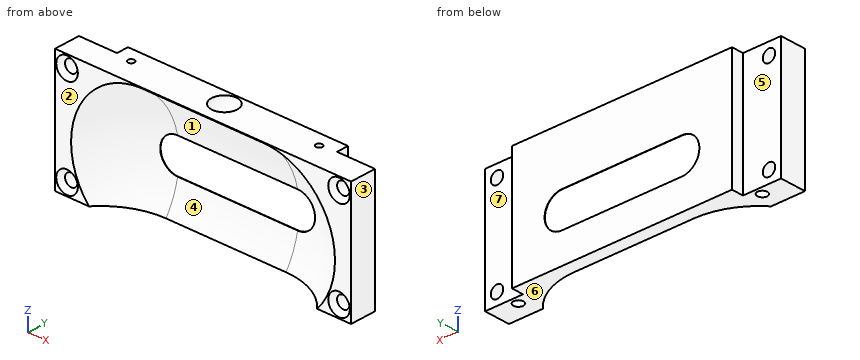
from build123d import *

# Parameters (mm, degrees)
SKETCH1_W                                       = 74
SKETCH1_H                                       = 30
BOSS_EXTRUDE1_DEPTH                             = 9.5
SKETCH2_W                                       = 9.5
SKETCH2_H                                       = 30
CUT_EXTRUDE1_DEPTH                              = 3
CSK_FOR_M3_FLAT_HEAD_MACHINE_SCREW1_D           = 3.1
CSK_FOR_M3_FLAT_HEAD_MACHINE_SCREW1_CSINK_D     = 5.4
CSK_FOR_M3_FLAT_HEAD_MACHINE_SCREW1_CSINK_ANGLE = 90
SKETCH14_W                                      = 30
SKETCH14_H                                      = 21.35
SKETCH21_R                                      = 0.8
CUT_EXTRUDE2_DEPTH                              = 6
TAP_DRILL_FOR_M3X0_5_TAP1_D                     = 2.5
TAP_DRILL_FOR_M3X0_5_TAP1_DEPTH                 = 4.5
TAP_DRILL_FOR_M3X0_5_TAP1_TIP                   = 0.751075774
CUT_EXTRUDE3_DEPTH                              = 10


with BuildPart() as part:
    # Sketch1 → Boss-Extrude1 (new body)
    with BuildSketch(Plane(origin=(0, 0, 0), x_dir=(1, 0, 0), z_dir=(0, 1, 0))):
        with Locations((37, 15)):
            Rectangle(SKETCH1_W, SKETCH1_H)
    extrude(amount=BOSS_EXTRUDE1_DEPTH)

    # Sketch2 → Cut-Extrude1 (cut)
    with BuildSketch(Plane(origin=(0, 9.5, 0), x_dir=(1, 0, 0), z_dir=(0, 1, 0))):
        with Locations((69.25, 15)):
            Rectangle(SKETCH2_W, SKETCH2_H)
        with Locations((4.75, 15)):
            Rectangle(SKETCH2_W, SKETCH2_H)
    extrude(amount=-CUT_EXTRUDE1_DEPTH, mode=Mode.SUBTRACT)

    # CSK for M3 Flat Head Machine Screw1 (through all)
    with Locations(Plane(origin=(3, 0, -3), x_dir=(0, 0, -1), z_dir=(0, -1, 0))):
        with Locations((0, 0), (24, 0), (24, 68), (0, 68)):
            CounterSinkHole(CSK_FOR_M3_FLAT_HEAD_MACHINE_SCREW1_D / 2, CSK_FOR_M3_FLAT_HEAD_MACHINE_SCREW1_CSINK_D / 2, counter_sink_angle=CSK_FOR_M3_FLAT_HEAD_MACHINE_SCREW1_CSINK_ANGLE)

    # Sketch12 → Cut-Revolve5 (revolve, cut)
    with BuildSketch(Plane(origin=(0, -11.5, 0), x_dir=(-1, 0, 0), z_dir=(0, -1, 0))):
        with BuildLine():
            Line((-52, -3.2), (-52, 39.5))
            ThreePointArc((-52, 39.5), (-73.35, 18.15), (-52, -3.2))
        make_face()
    revolve(axis=Axis((52, -11.5, 3.2), (0, 0, -1)), mode=Mode.SUBTRACT)

    # Sketch12<8> → Cut-Revolve6 (revolve, cut)
    with BuildSketch(Plane(origin=(0, -11.5, 0), x_dir=(-1, 0, 0), z_dir=(0, -1, 0))):
        with BuildLine():
            Line((-22, -3.2), (-22, 39.5))
            ThreePointArc((-22, 39.5), (-0.65, 18.15), (-22, -3.2))
        make_face()
    revolve(axis=Axis((22, -11.5, 3.2), (0, 0, -1)), mode=Mode.SUBTRACT)

    # Sketch14 → Cut-Revolve7 (revolve, cut)
    with BuildSketch(Plane(origin=(0, -11.5, 0), x_dir=(-1, 0, 0), z_dir=(0, -1, 0))):
        with Locations((-37, 28.825)):
            Rectangle(SKETCH14_W, SKETCH14_H)
    revolve(axis=Axis((52, -11.5, -18.15), (-1, 0, 0)), mode=Mode.SUBTRACT)

    # Sketch20 one side → Cut-Revolve8 (revolve, cut)
    with BuildSketch(Plane.XY):
        with BuildLine():
            ThreePointArc((37, 9), (33.8, 5.8), (37, 2.6))
            Line((37, 2.6), (37, 9))
        make_face()
    revolve(axis=Axis((37, 9, 0), (0, -1, 0)), mode=Mode.SUBTRACT)

    # Sketch21 → Cut-Extrude2 (cut)
    with BuildSketch(Plane.XY):
        with Locations((13.5, 6)):
            Circle(SKETCH21_R)
        with Locations((60.5, 6)):
            Circle(SKETCH21_R)
    extrude(amount=-CUT_EXTRUDE2_DEPTH, mode=Mode.SUBTRACT)

    # Tap Drill for M3x0.5 Tap1
    with Locations(Plane(origin=(6.5, 4.5, -30), x_dir=(-1, 0, 0), z_dir=(0, 0, -1))):
        with Locations((0, 0), (-61, 0)):
            Hole(TAP_DRILL_FOR_M3X0_5_TAP1_D / 2, depth=TAP_DRILL_FOR_M3X0_5_TAP1_DEPTH)
            with Locations((0, 0, -(TAP_DRILL_FOR_M3X0_5_TAP1_DEPTH + TAP_DRILL_FOR_M3X0_5_TAP1_TIP / 2))):  # 118° drill point
                Cone(0, TAP_DRILL_FOR_M3X0_5_TAP1_D / 2, TAP_DRILL_FOR_M3X0_5_TAP1_TIP, mode=Mode.SUBTRACT)

    # Sketch26 → Cut-Extrude3 (cut)
    with BuildSketch(Plane(origin=(0, 9.5, 0), x_dir=(1, 0, 0), z_dir=(0, 1, 0))):
        with BuildLine():
            Line((52, 13.8), (22, 13.8))
            ThreePointArc((22, 13.8), (17.65, 18.15), (22, 22.5))
            Line((22, 22.5), (52, 22.5))
            ThreePointArc((52, 22.5), (56.35, 18.15), (52, 13.8))
        make_face()
    extrude(amount=-CUT_EXTRUDE3_DEPTH, mode=Mode.SUBTRACT)


solid = part.part
Part model, mm, in its own coordinate system. Face numbers are marked on the shaded views. A direction names the side the tool comes from. Give positions to 0.01 mm unless a question says otherwise; leave off trailing zeros. Order: outer loops, then holes, each group sorted by start corner. A loop starts at its lowest first (then second) coordinate and runs counter-clockwise, first axis right, second up. Notation, with made-up numbers: (24, -21.75) -> (78, -21.75) arc R12 ccw to (78, -2.75) -> close; hole circle Ø1 at (39.25, -18.75). An arc over 180 degrees is marked (long way). Use one line per item in the form item = value.
(1) Saw through at D-D (z = -9). Write the cut outline in (x, y).
Solution:
outline = (0, 0) -> (6.51, 0) arc R19.29 cw to (22, 7.79) -> (52, 7.79) arc R19.29 cw to (67.49, 0) -> (74, 0) -> (74, 6.5) -> (64.5, 6.5) -> (64.5, 9.5) -> (9.5, 9.5) -> (9.5, 6.5) -> (0, 6.5) -> close
(2) Flat gauge pins, fed straight in: P1, Ø4, axis at x = 3, z = -27, coming from the -Y side; P2, Ø1.3, axis at x = 61, y = 5.5, coming from the +Z side; P3, Ø1, axis at x = 35, z = -12.5, coming from the -Y side; P4, Ø10.5, axis at x = 70.5, z = -17, coming from the +Y side. Where does each tip first touch, or does it go through?
Solution:
P1 = 0.7
P2 = 0
P3 = 8.95
P4 = 6.5
(3) Pull direction X, two halves, no side cores. Call the marked faces 1, 2, 3 and 4: +X half, -X half, draft (parallel to the pull), parting line (faces both ways), or undercut.
Solution:
face_1 = undercut
face_2 = draft
face_3 = +X half
face_4 = undercut
(4) Drill centre lines: line 1 (Z direction, x = 3, y = 5.4); line 2 (Y direction, x = 67.5, z = -29); line 3 (X direction, y = 4.5, z = -27.5). Where is each one in solid material? Low to high. Write a range as from..to.
Solution:
line_1 = -30..-28.55, -25.45..-4.55, -1.45..0
line_2 = 0..3.25, 5.75..6.5
line_3 = 0..1.53, 4.47..5.25, 7.75..11.4, 62.6..66.25, 68.75..69.53, 72.47..74
(5) Tool access for the marked faces 5, 6 and 7: list every direction of +Z, -Z, +X, -X, +Y, -Y with a clear straight run to the whole face (end or side of a thin tool).
Solution:
face_5 = +Z, -Z, -X, +Y
face_6 = -Z, +X, -X, +Y, -Y
face_7 = +Z, -Z, +X, +Y
(6) Saw through at B-B (x = 71). Write the cut outline in (y, z), then the cut area to 3 significant figures.
Solution:
outline = (0, -30) -> (6.5, -30) -> (6.5, -28.55) -> (1.15, -28.55) -> (0, -29.7) -> close; (0, -24.3) -> (1.15, -25.45) -> (6.5, -25.45) -> (6.5, -4.55) -> (1.15, -4.55) -> (0, -5.7) -> close; (0, -0.3) -> (1.15, -1.45) -> (6.5, -1.45) -> (6.5, 0) -> (0, 0) -> close
area = 152 mm²
(7) Saw through at C-C (x = 48). Write the cut outline in (y, z), then the cut area to 3 significant figures.
Solution:
outline = (0, -0.16) arc R21.35 cw to (9.4, -13.8) -> (9.5, -13.8) -> (9.5, 0) -> (0, 0) -> close; (6.26, -30) -> (9.5, -30) -> (9.5, -22.5) -> (9.4, -22.5) arc R21.35 cw to start
area = 58.8 mm²
(8) Saw through at A-A (z = -18.15). Write the cut outline in (x, y).
Solution:
outline = (0, 0) -> (4.01, 0) arc R21.35 cw to (17.65, 9.4) -> (17.65, 9.5) -> (9.5, 9.5) -> (9.5, 6.5) -> (0, 6.5) -> close; (56.35, 9.4) arc R21.35 cw to (69.99, 0) -> (74, 0) -> (74, 6.5) -> (64.5, 6.5) -> (64.5, 9.5) -> (56.35, 9.5) -> close
